from build123d import *

# Parameters (mm, degrees)
SKETCH1_W           = 29
SKETCH1_H           = 44
BOSS_EXTRUDE1_DEPTH = 2
SKETCH2_W           = 29
SKETCH2_H           = 44
BOSS_EXTRUDE2_DEPTH = 5
CUT_EXTRUDE1_DEPTH  = 45.980551353
CUT_EXTRUDE2_DEPTH  = 39.93906297
SKETCH8_R           = 1.5
BOSS_EXTRUDE3_DEPTH = 5
FILLET1_R           = 1


with BuildPart() as part:
    # Sketch1 → Boss-Extrude1 (new body)
    with BuildSketch(Plane.XY):
        with Locations((0, 3.025)):
            Rectangle(SKETCH1_W, SKETCH1_H)
    extrude(amount=BOSS_EXTRUDE1_DEPTH)

    # Sketch2 → Boss-Extrude2 (add)
    with BuildSketch(Plane.XY.offset(2)):
        with Locations((0, 3.025)):
            Rectangle(SKETCH2_W, SKETCH2_H)
        Polygon((12.5, 23.025), (12.5, 16.975), (12.5, -16.975), (-12.5, -16.975), (-12.5, 16.975), (-12.5, 23.025), align=None, mode=Mode.SUBTRACT)
    extrude(amount=BOSS_EXTRUDE2_DEPTH)

    # Sketch4 → Cut-Extrude1 (cut, through all)
    with BuildSketch(Plane(origin=(0, -16.975, 0), x_dir=(1, 0, 0), z_dir=(0, 1, 0))):
        with BuildLine():
            Line((-2.5, -7), (2.5, -7))
            ThreePointArc((2.5, -7), (0, -4.5), (-2.5, -7))
        make_face()
    extrude(amount=-CUT_EXTRUDE1_DEPTH, mode=Mode.SUBTRACT)

    # Sketch5 → Cut-Extrude2 (cut, through all)
    with BuildSketch(Plane.ZY.offset(14.5)):
        Polygon((5, 5.525), (5, 0.525), (4.5, 0.525), (2.5, 0.525), (2.5, 5.525), (4.5, 5.525), align=None)
    extrude(amount=-CUT_EXTRUDE2_DEPTH, mode=Mode.SUBTRACT)

    # Sketch8 → Boss-Extrude3 (add)
    with BuildSketch(Plane.XY.offset(2)):
        with Locations((-7.625, 19.775)):
            Circle(SKETCH8_R)
        with Locations(Location((-7.625, -7.675, 0), (0, 0, 180))):
            Circle(SKETCH8_R)
        with Locations((7.625, -7.675)):
            Circle(SKETCH8_R)
        with Locations(Location((7.625, 19.775, 0), (0, 0, 180))):
            Circle(SKETCH8_R)
    extrude(amount=BOSS_EXTRUDE3_DEPTH)

    # Fillet1
    # the kernel refuses this fillet: 1 mm, written as the material it adds along each edge
    with BuildSketch(Plane(origin=(12.5, 23.025, 2), x_dir=(0, 0, 1), z_dir=(0, -1, 0))) as fillet1_piece_1_section:
        with BuildLine():
            CenterArc((FILLET1_R, FILLET1_R), FILLET1_R, 180, 90)
            Line((0, FILLET1_R), (0, 0))
            Line((0, 0), (FILLET1_R, 0))
        make_face()
    fillet1_piece_1 = extrude(amount=42.5, mode=Mode.PRIVATE)
    fillet1_piece_1 = split(fillet1_piece_1, bisect_by=Plane(origin=(12.460315407, 5.525, 2.623263613), z_dir=(0, 1, 0)), keep=Keep.TOP, mode=Mode.PRIVATE)
    add(fillet1_piece_1)
    with BuildSketch(Plane(origin=(12.5, 25.525, 2), x_dir=(0, 0, 1), z_dir=(0, -1, 0))) as fillet1_piece_2_section:
        with BuildLine():
            CenterArc((FILLET1_R, FILLET1_R), FILLET1_R, 180, 90)
            Line((0, FILLET1_R), (0, 0))
            Line((0, 0), (FILLET1_R, 0))
        make_face()
    fillet1_piece_2 = extrude(amount=42.5, mode=Mode.PRIVATE)
    fillet1_piece_2 = split(fillet1_piece_2, bisect_by=Plane(origin=(12.255975151, 3.025, 2.5), z_dir=(0, 0, -1)), keep=Keep.TOP, mode=Mode.PRIVATE)
    fillet1_piece_2 = split(fillet1_piece_2, bisect_by=Plane(origin=(12.255975151, 5.525, 2.17839593), z_dir=(0, -1, 0)), keep=Keep.TOP, mode=Mode.PRIVATE)
    add(fillet1_piece_2)
    with BuildSketch(Plane(origin=(12.5, 25.525, 2), x_dir=(0, 0, 1), z_dir=(0, -1, 0))) as fillet1_piece_3_section:
        with BuildLine():
            CenterArc((FILLET1_R, FILLET1_R), FILLET1_R, 180, 90)
            Line((0, FILLET1_R), (0, 0))
            Line((0, 0), (FILLET1_R, 0))
        make_face()
    fillet1_piece_3 = extrude(amount=42.5, mode=Mode.PRIVATE)
    fillet1_piece_3 = split(fillet1_piece_3, bisect_by=Plane(origin=(12.460315407, 0.525, 2.623263613), z_dir=(0, -1, 0)), keep=Keep.TOP, mode=Mode.PRIVATE)
    add(fillet1_piece_3)
    # the kernel refuses this fillet: 1 mm, written as the material it takes off along each edge
    with BuildSketch(Plane(origin=(13.5, 24.025, 1), x_dir=(0, 0, -1), z_dir=(0, 1, 0))) as fillet1_2_piece_1_section:
        Polygon((0, 0), (FILLET1_R * 1.02, 0), (FILLET1_R * 1.02, -FILLET1_R * 1.02), (0, -FILLET1_R * 1.02), align=None)
    fillet1_2_piece_1 = extrude(amount=FILLET1_R * 1.02, mode=Mode.PRIVATE)
    fillet1_2_piece_1 = fillet1_2_piece_1 - Plane(origin=(13.5, 24.025, 1), x_dir=(-0.7071067811865475, 0, 0.7071067811865475), z_dir=(0, 1, 0)) * Sphere(FILLET1_R, mode=Mode.PRIVATE)
    add(fillet1_2_piece_1, mode=Mode.SUBTRACT)
    with BuildSketch(Plane(origin=(13.5, -17.975, 1), x_dir=(1, 0, 0), z_dir=(0, 0, -1))) as fillet1_2_piece_2_section:
        Polygon((0, 0), (FILLET1_R * 1.02, 0), (FILLET1_R * 1.02, FILLET1_R * 1.02), (0, FILLET1_R * 1.02), align=None)
    fillet1_2_piece_2 = extrude(amount=FILLET1_R * 1.02, mode=Mode.PRIVATE)
    fillet1_2_piece_2 = fillet1_2_piece_2 - Plane(origin=(13.5, -17.975, 1), x_dir=(-0.7071067811865476, 0.7071067811865475, 0), z_dir=(0, 0, -1)) * Sphere(FILLET1_R, mode=Mode.PRIVATE)
    add(fillet1_2_piece_2, mode=Mode.SUBTRACT)
    with BuildSketch(Plane(origin=(-13.5, -17.975, 1), x_dir=(0, -1, 0), z_dir=(0, 0, -1))) as fillet1_2_piece_3_section:
        Polygon((0, 0), (FILLET1_R * 1.02, 0), (FILLET1_R * 1.02, FILLET1_R * 1.02), (0, FILLET1_R * 1.02), align=None)
    fillet1_2_piece_3 = extrude(amount=FILLET1_R * 1.02, mode=Mode.PRIVATE)
    fillet1_2_piece_3 = fillet1_2_piece_3 - Plane(origin=(-13.5, -17.975, 1), x_dir=(0.7071067811865475, 0.7071067811865477, 0), z_dir=(0, 0, -1)) * Sphere(FILLET1_R, mode=Mode.PRIVATE)
    add(fillet1_2_piece_3, mode=Mode.SUBTRACT)
    with BuildSketch(Plane(origin=(-13.5, 24.025, 1), x_dir=(0, 0, -1), z_dir=(0, 1, 0))) as fillet1_2_piece_4_section:
        Polygon((0, 0), (FILLET1_R * 1.02, 0), (FILLET1_R * 1.02, FILLET1_R * 1.02), (0, FILLET1_R * 1.02), align=None)
    fillet1_2_piece_4 = extrude(amount=FILLET1_R * 1.02, mode=Mode.PRIVATE)
    fillet1_2_piece_4 = fillet1_2_piece_4 - Plane(origin=(-13.5, 24.025, 1), x_dir=(0.7071067811865475, 0, 0.7071067811865475), z_dir=(0, 1, 0)) * Sphere(FILLET1_R, mode=Mode.PRIVATE)
    add(fillet1_2_piece_4, mode=Mode.SUBTRACT)
    with BuildSketch(Plane(origin=(14.5, 24.025, 0), x_dir=(-1, 0, 0), z_dir=(0, -1, 0)), Plane(origin=(-14.5, -17.975, 0), x_dir=(1, 0, 0), z_dir=(0, 1, 0))) as fillet1_2_piece_5:
        with BuildLine():
            CenterArc((FILLET1_R, -FILLET1_R), FILLET1_R, 90, 90)
            Line((0, -FILLET1_R), (0, 0))
            Line((0, 0), (FILLET1_R, 0))
        make_face()
    extrude(amount=42, mode=Mode.SUBTRACT)
    with BuildSketch(Plane(origin=(13.5, -18.975, 0), x_dir=(0, 1, 0), z_dir=(-1, 0, 0))) as fillet1_2_piece_6:
        with BuildLine():
            CenterArc((FILLET1_R, -FILLET1_R), FILLET1_R, 90, 90)
            Line((0, -FILLET1_R), (0, 0))
            Line((0, 0), (FILLET1_R, 0))
        make_face()
    extrude(amount=27, mode=Mode.SUBTRACT)
    with BuildSketch(Plane(origin=(14.5, -18.975, 9.5), x_dir=(-1, 0, 0), z_dir=(0, 0, -1)), Plane(origin=(-14.5, -18.975, 1), x_dir=(1, 0, 0), z_dir=(0, 0, 1))) as fillet1_2_piece_7:
        with BuildLine():
            CenterArc((FILLET1_R, FILLET1_R), FILLET1_R, 180, 90)
            Line((0, FILLET1_R), (0, 0))
            Line((0, 0), (FILLET1_R, 0))
        make_face()
    extrude(amount=8.5, mode=Mode.SUBTRACT)
    with BuildSketch(Plane(origin=(-14.5, 25.025, 1), x_dir=(1, 0, 0), z_dir=(0, 0, 1)), Plane(origin=(14.5, 25.025, 9.5), x_dir=(-1, 0, 0), z_dir=(0, 0, -1))) as fillet1_2_piece_8:
        with BuildLine():
            CenterArc((FILLET1_R, -FILLET1_R), FILLET1_R, 90, 90)
            Line((0, -FILLET1_R), (0, 0))
            Line((0, 0), (FILLET1_R, 0))
        make_face()
    extrude(amount=8.5, mode=Mode.SUBTRACT)
    with BuildSketch(Plane(origin=(-13.5, 25.025, 0), x_dir=(0, 0, 1), z_dir=(1, 0, 0))) as fillet1_2_piece_9:
        with BuildLine():
            CenterArc((FILLET1_R, FILLET1_R), FILLET1_R, 180, 90)
            Line((0, FILLET1_R), (0, 0))
            Line((0, 0), (FILLET1_R, 0))
        make_face()
    extrude(amount=27, mode=Mode.SUBTRACT)


solid = part.part
Part model, mm, in its own coordinate system. A direction names the side the tool comes from. Coordinates: 2 decimals unless noted, no trailing zeros. Write each loop counter-clockwise with the first axis right and the second up, starting at its lowest first coordinate (ties: lowest second). Pieces come first, ordered by that corner, then holes. Notation, with made-up numbers: M 8,-16 L 46,-16 A19 ccw 46,-2 Z; hole C 55,45.25 d7. An arc over 180 degrees is marked long. Return JSON: item names as keys, results as strings.
1. 3-axis set-ups, long thin cutter, end or side, ignore diameter. For faces 1 (the face through (0, -16.975, 4)), 2 (the face through (13, 5.525, 4)), 3 (the face through (-14.5, 2.7, 5.3)): which of +Z, -Z, +X, -X, +Y, -Y reach the whole face in a straight line?
Determined:
{"face 1": "+Z", "face 2": "+X, -X", "face 3": "+Z, -Z, -X, +Y, -Y"}
2. Saw through at A-A, the plane x = -3. Write the cut outline in (y, z) (3 decimals), then the cut area to 3 significant figures.
Determined:
{"outline": "M -18.975,1 A1 ccw -17.975,0 L 24.025,0 A1 ccw 25.025,1 L 25.025,7 L 23.025,7 L 23.025,2 L -16.975,2 L -16.975,7 L -18.975,7 Z", "area": "108 mm²"}
3. Probe L1, parallel to Z at x = -13, y = 3; L2, parallel to Y at x = -12.25, z = 5.5 (3 decimals); L3, parallel to X at y = -15.5, z = 4.5. List the from-to ranges inside material, lowest first.
Determined:
{"L1": "0 to 2.5, 5 to 7", "L2": "-18.975 to -16.975, 23.025 to 25.025", "L3": "-14.5 to -12.5, 12.5 to 14.5"}
4. Pull direction X, two halves, no side cores. Call faces 4 (the face through (0.1, -18, 4.5)), 5 (the face through (13, 3, 5)), 6 (the face through (-14.2, 24.74, 3.96)), 7 (the face through (14.2, 24.74, 4.04)): pulls with the +X half, pulls with the -X half, needs draft (parallel to the pull), parting line crosses it, or undercut.
Determined:
{"face 4": "undercut", "face 5": "needs draft", "face 6": "pulls with the -X half", "face 7": "pulls with the +X half"}
5. Saw through at B-B, the plane z = 3.5. Write the cut outline in (x, y) (3 decimals).
Determined:
{"outline": "M -14.5,-17.975 A1 ccw -13.5,-18.975 L 13.5,-18.975 A1 ccw 14.5,-17.975 L 14.5,0.525 L 12.5,0.525 L 12.5,-16.975 L -12.5,-16.975 L -12.5,0.525 L -14.5,0.525 Z; M -14.5,5.525 L -12.5,5.525 L -12.5,23.025 L 12.5,23.025 L 12.5,5.525 L 14.5,5.525 L 14.5,24.025 A1 ccw 13.5,25.025 L -13.5,25.025 A1 ccw -14.5,24.025 Z; C -7.625,-7.675 d3; C -7.625,19.775 d3; C 7.625,-7.675 d3; C 7.625,19.775 d3"}
6. Saw through at D-D, the plane x = 0. Write the cut outline in (y, z) (3 decimals), then the cut area to 3 significant figures.
Determined:
{"outline": "M -18.975,1 A1 ccw -17.975,0 L 24.025,0 A1 ccw 25.025,1 L 25.025,7 L 23.025,7 L 23.025,2 L -16.975,2 L -16.975,4.5 L -18.975,4.5 Z", "area": "103 mm²"}
7. Flat gauge pin, fed straight in: pin 1 Ø2 at (x, y) = (6, 1) entering from +Z. Where does the tip first touch, or does it go through?
Determined:
{"pin 1": "z = 2"}
8. Saw through at C-C, the plane y = -0.5. Write the cut outline in (x, z), then the cut area to 3 significant figures.
Determined:
{"outline": "M -14.5,1 A1 ccw -13.5,0 L 13.5,0 A1 ccw 14.5,1 L 14.5,7 L 12.5,7 L 12.5,3 A1 cw 11.5,2 L -12.5,2 L -12.5,7 L -14.5,7 Z", "area": "77.8 mm²"}
